Here's how the part is built. I have some questions about the finished solid (model axes, mm). Face numbers are marked on the shaded views. A direction names the side the tool comes from. Round coordinates to 2 decimals unless told otherwise and drop trailing zeros. Order: outer loops, then holes, each group sorted by start corner. A loop starts at its lowest first (then second) coordinate and runs counter-clockwise, first axis right, second up. Notation, with made-up numbers: M 89,-37.5 L 135,-37.5 A27 ccw 135,-15.5 Z; hole C 72,9 d4. An arc over 180 degrees is marked long. Write item = value, one per line. Start each with the question number.
Item 1: I want a section at A-A, the plane z = 0. List the corners of the cut face in (x, y) for me, plus the area to 3 significant figures.
Item 2: I want a section at B-B, the plane y = -6. List the corners of the cut face in (x, z) for me.
Item 3: I want a section at C-C, the plane x = 0. List the corners of the cut face in (y, z) for me.
Item 4: We'd pull the mould along X, two halves only. Please class the marked faces 4, 5 and 6: pulls with the +X half, pulls with the -X half, needs draft (parallel to the pull), parting line crosses it, or undercut.
Item 5: For the marked faces 1, 2 and 3, which set-ups out of +Z, -Z, +X, -X, +Y, -Y let a thin tool reach every point of the face, with its end or its side?
Item 6: I'm going to push flat-ended pins straight in: P1, Ø1.8, axis at y = -6.5, z = 20.5, coming from the +X side; P2, Ø2.5, axis at y = -6.5, z = 20.5, coming from the -X side; P3, Ø1.5, axis at y = -4, z = -11.5, coming from the -X side. Where does each tip first touch, or does it pass through?
Item 7: Please list where these lines run through material, in increasing order: L1, parallel to Z at x = 0, y = -7.5; L2, parallel to Z at x = 5.5, y = -9.75; L3, parallel to X at y = -8.25, z = 6.
Item 8: I want a section at D-D, the plane y = -1.5. List the corners of the cut face in (x, z) for me, plus the area to 3 significant figures.
```python
from build123d import *

# Parameters (mm, degrees)
F0_R     = 13.67397
F1_DEPTH = 11.5
F2_W     = 7.456396
F2_H     = 4.709303
F3_DEPTH = 7.3
F4_R     = 2.5


with BuildPart() as f1:
    # F0 (on Front) → F1 (new body)
    with BuildSketch(Plane.XZ):
        with BuildLine():
            Line((-19.229384, 1.655212), (-19.229384, -1.655212))
            ThreePointArc((-19.229384, -1.655212), (-4.219579, -18.833589), (16.684931, -9.701649))
            Line((16.684931, -9.701649), (16.684931, 9.701649))
            ThreePointArc((16.684931, 9.701649), (13.647508, 13.647508), (9.701649, 16.684931))
            Line((9.701649, 16.684931), (-9.701649, 16.684931))
            ThreePointArc((-9.701649, 16.684931), (-16.301052, 10.333665), (-19.229384, 1.655212))
        make_face()
        Circle(F0_R, mode=Mode.SUBTRACT)
    extrude(amount=F1_DEPTH)

    # F2 (on face) → F3 (join)
    with BuildSketch(Plane.XY.offset(16.684931)):
        with Locations((0, -6.213662)):
            Rectangle(F2_W, F2_H)
    extrude(amount=F3_DEPTH)

    # F4
    f4_edges = [f1.edges().sort_by_distance(p)[0] for p in [
        (-3.728198, -6.213663, 23.984931),
        (3.728198, -6.213663, 23.984931),
        (3.728198, -6.213663, 16.684931),
        (-3.728198, -6.213663, 16.684931),
    ]]
    fillet(f4_edges, radius=F4_R)


solid = f1.part
```
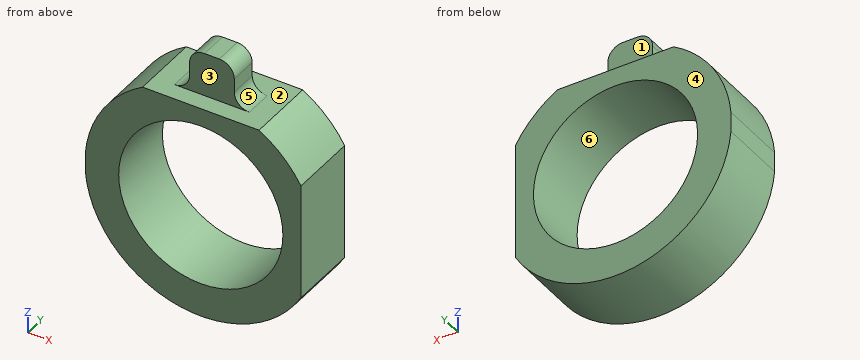
Filled in:
q1.outline = M -19.23,-11.5 L -13.67,-11.5 L -13.67,0 L -19.23,0 Z; M 13.67,-11.5 L 16.68,-11.5 L 16.68,0 L 13.67,0 Z
q1.area = 98.5 mm^2
q2.outline = M -19.23,-1.66 A19.3 ccw 16.68,-9.7 L 16.68,9.7 A19.3 ccw 9.7,16.68 L 6.23,16.68 A2.5 cw 3.73,19.18 L 3.73,21.48 A2.5 ccw 1.23,23.98 L -1.23,23.98 A2.5 ccw -3.73,21.48 L -3.73,19.18 A2.5 cw -6.23,16.68 L -9.7,16.68 A19.3 ccw -19.23,1.66 Z; hole C 0,0 d27.35
q3.outline = M -11.5,-19.3 L 0,-19.3 L 0,-13.67 L -11.5,-13.67 Z; M -11.5,13.67 L 0,13.67 L 0,16.68 L -3.86,16.68 L -3.86,23.98 L -8.57,23.98 L -8.57,16.68 L -11.5,16.68 Z
q4.face_4 = needs draft
q4.face_5 = pulls with the +X half
q4.face_6 = undercut
q5.face_1 = +Z, +X, -X, +Y
q5.face_2 = +Z
q5.face_3 = +Z, +X, -X, -Y
q6.P1 = 3.73
q6.P2 = -3.73
q6.P3 = -16.03
q7.L1 = -19.3 to -13.67, 13.67 to 23.98
q7.L2 = -18.5 to -12.52, 12.52 to 16.68
q7.L3 = -18.34 to -12.29, 12.29 to 16.68
q8.outline = M -19.23,-1.66 A19.3 ccw 16.68,-9.7 L 16.68,9.7 A19.3 ccw 9.7,16.68 L -9.7,16.68 A19.3 ccw -19.23,1.66 Z; hole C 0,0 d27.35
q8.area = 514 mm^2
